Input: part model. Units: mm. Frame: model coordinates. A direction names the side the tool comes from. Give positions to 0.01 mm unless a question says otherwise; leave off trailing zeros. Loops run counter-clockwise (first coordinate to the right, second up) from the corner with the lowest first, then second, coordinate; pieces in that order, holes last. Notation, with made-up numbers: (-1, -14) -> (18, -14) arc R10 ccw to (18, 0) -> close; hole circle Ø11 at (16.25, -13.75). An arc over 180 degrees is marked (long way). Answer as a JSON object with one key per item and string values. Group by question number.
```python
from build123d import *

# Parameters (mm, degrees)
SKETCH_1_R                  = 4
EXTRUDE_1_DEPTH             = 37
SKETCH_2_R                  = 4
SKETCH_2_R_2                = 3.9
SKETCH_2_R_3                = 0.5
CUT_EXTRUDE_1_DEPTH         = 1
CUT_EXTRUDE_2_DEPTH         = 38.429934544
CUT_EXTRUDE_2_DEPTH_BACK    = 38.429934544
EXTRUDE_2_REACH             = 39.43
SKETCH_4_R                  = 1.9
EXTRUDE_2_DIRECTION_2_DEPTH = 5


with BuildPart() as part:
    # Sketch 1 → Extrude 1 (new body)
    with BuildSketch(Plane.XY):
        Circle(SKETCH_1_R)
    extrude(amount=EXTRUDE_1_DEPTH)

    # Sketch 2 → Cut-Extrude 1 (cut)
    # profile 1 of 2: a face of its own
    with BuildSketch(Plane(origin=(0, 0, 0), x_dir=(-1, 0, 0), z_dir=(0, 0, -1))):
        Circle(SKETCH_2_R)
        Circle(SKETCH_2_R_2, mode=Mode.SUBTRACT)
    # profile 2 of 2: a face of its own
    with BuildSketch(Plane(origin=(0, 0, 0), x_dir=(-1, 0, 0), z_dir=(0, 0, -1))):
        Circle(SKETCH_2_R_3)
    extrude(amount=-CUT_EXTRUDE_1_DEPTH, mode=Mode.SUBTRACT)

    # Sketch 3 → Cut-Extrude 2 (cut, two sides: drawn at the far end of the back side and taken through both)
    with BuildSketch(Plane(origin=(0, 0, 0), x_dir=(1, 0, 0), z_dir=(0, 1, 0)).offset(-CUT_EXTRUDE_2_DEPTH_BACK)):
        with BuildLine():
            Line((-3, -37), (4, -37))
            Line((4, -37), (4, -34))
            ThreePointArc((4, -34), (0.807886553, -36.218401957), (-3, -37))
        make_face()
    extrude(amount=CUT_EXTRUDE_2_DEPTH + CUT_EXTRUDE_2_DEPTH_BACK, mode=Mode.SUBTRACT)

    # Sketch 4 → Extrude 2 (add, up to next)
    with BuildSketch(Plane.XY.offset(37), mode=Mode.PRIVATE) as extrude_2_sk1:
        with Locations(Location((-2, 0, 0), (0, 0, 238.243136141))):
            Circle(SKETCH_4_R)
    extrude_2_tool1 = extrude(extrude_2_sk1.sketch, amount=-EXTRUDE_2_REACH, mode=Mode.PRIVATE) - part.part
    add(extrude_2_tool1.solids().sort_by_distance((-2, 0, 37))[0])

    # Sketch 4 → Extrude 2 direction 2 (add)
    with BuildSketch(Plane.XY.offset(37)):
        with Locations(Location((-2, 0, 0), (0, 0, 238.243136141))):
            Circle(SKETCH_4_R)
    extrude(amount=EXTRUDE_2_DIRECTION_2_DEPTH)


solid = part.part
```
Q1. Ray query, probe 1 along Y at (x, z) = (0, 0.45); probe 2 along Y at (x, z) = (0.25, 26.5); probe 3 along Y at (x, z) = (3, 18). Return the intervals inside material, ascending.
Q2. Set-up query: faces 4 (the face through (-4, 0, 19)), 5 (the face through (-0.17, 0.51, 39.24)), 6 (the face through (0, 0, 1)). Return all of +Z, -Z, +X, -X, +Y, -Y with unobstructed straight access to the full face (end or side cutting, diameter ignored); none if empty.
Q3. Pull-direction query (X, two-part tool) for faces 1 (the face through (0.108, -0.488, 0.493)), 2 (the face through (-2, 0, 42)), 3 (the face through (2.87, 2.64, 0.49)); classes: +X half, -X half, draft (parallel to the pull), parting line (faces both ways), or undercut.
Q4. Section B-B on z = 25. Return the cut outline in (x, y).
Q5. Section A-A on x = -3.5. Return the cut outline in (y, z), then the cut area to 3 significant figures.
Q6. Section C-C on x = -1.75. Return the cut outline in (y, z), then the cut area to 3 significant figures.
Q7. Section D-D on z = 39. Return the cut outline in (x, y), then the cut area to 3 significant figures.
Q8. Pin query (flat end, axial travel): pin 1 Ø4 at (y, z) = (3, 35.5) entering from -X; pin 2 Ø1 at (x, z) = (2.5, 30) entering from -Y; pin 3 Ø1.5 at (y, z) = (1, 35) entering from +X. Return the tip coordinate at first contact, or that it passes through.
Numbers:
{
 "1": {"probe 1": "y = -3.9 to -0.5, 0.5 to 3.9", "probe 2": "y = -3.99 to 3.99", "probe 3": "y = -2.65 to 2.65"},
 "2": {"face 4": "+Z, -Z", "face 5": "+Z", "face 6": "-Z"},
 "3": {"face 1": "undercut", "face 2": "draft", "face 3": "parting line"},
 "4": {"outline": "circle Ø8 at (0, 0)"},
 "5": {"outline": "(-1.94, 1) -> (-1.72, 1) -> (-1.72, 0) -> (1.72, 0) -> (1.72, 1) -> (1.94, 1) -> (1.94, 37) -> (1.17, 37) -> (1.17, 42) -> (-1.17, 42) -> (-1.17, 37) -> (-1.94, 37) -> close", "area": "155 mm²"},
 "6": {"outline": "(-3.6, 1) -> (-3.49, 1) -> (-3.49, 0) -> (3.49, 0) -> (3.49, 1) -> (3.6, 1) -> (3.6, 36.92) -> (1.88, 36.92) -> (1.88, 42) -> (-1.88, 42) -> (-1.88, 36.92) -> (-3.6, 36.92) -> close", "area": "285 mm²"},
 "7": {"outline": "circle Ø3.8 at (-2, 0)", "area": "11.3 mm²"},
 "8": {"pin 1": "stops at x = -3.87", "pin 2": "stops at y = -3.46", "pin 3": "stops at x = 3.75"}
}
